Can you work these out from the drawing? Everything is in mm from the part's minimum corner. A direction names the side the tool comes from. Round coordinates to 2 decimals unless told otherwise and drop trailing zeros. Order: outer loops, then holes, each group sorted by start corner. A loop starts at its lowest first (then second) coordinate and runs counter-clockwise, first axis right, second up. Notation, with made-up numbers: (42.5, 17) -> (96.5, 17) arc R17 ccw to (96.5, 32) -> close; hole circle Ø7 at (15.25, 86.5). An arc over 180 degrees is marked (long way). One line per item, written item: value.
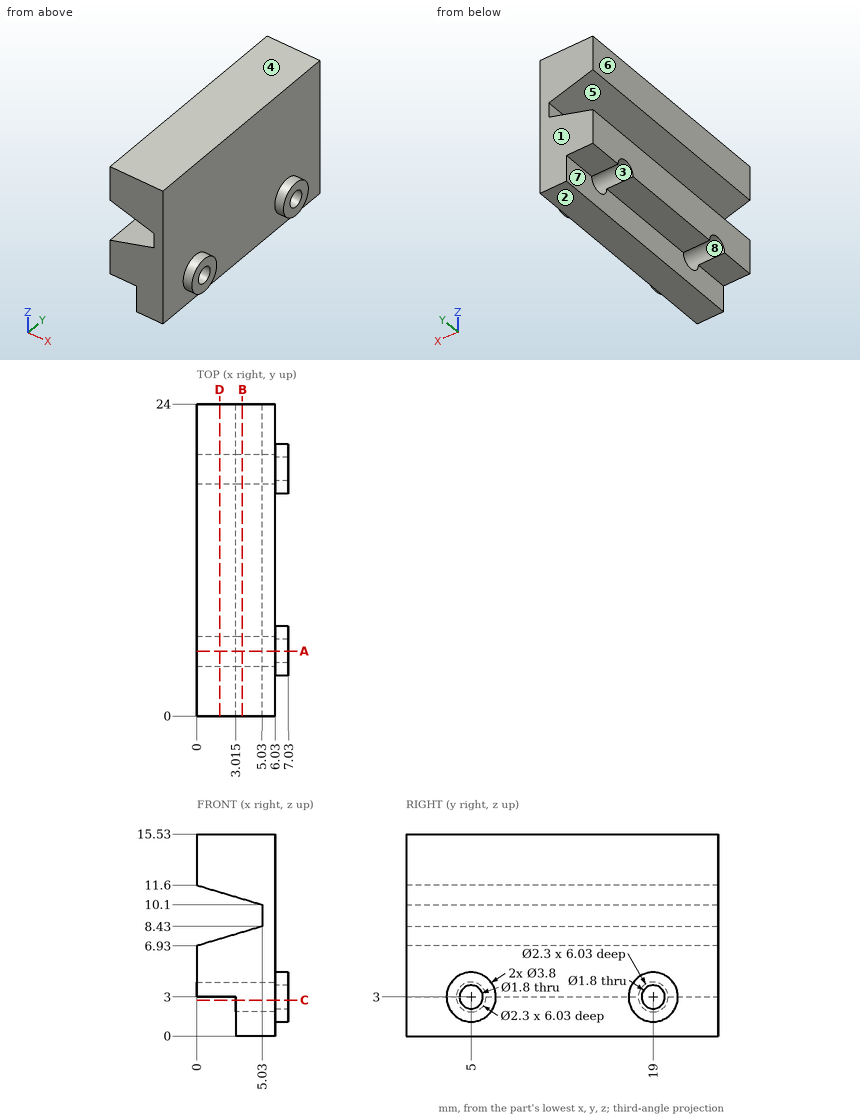
Q1. On a 3-axis mill with a long thin cutter (end or side, diameter ignored), from which of +Z, -Z, +X, -X, +Y, -Y can I reach the whole of each face in a straight line? I mean the marked faces 5, 6, 7 and 8. Say none if no direction works.
Answers below:
face 5: -X, +Y, -Y
face 6: +Z, -Z, -X, +Y, -Y
face 7: -Z, -X, +Y, -Y
face 8: -X
Q2. Will these pins go through, and if not, where does the flat tip stop? pin 1 Ø2 at (y, z) = (19, 3) entering from -X; pin 2 Ø1.4 at (y, z) = (5, 3) entering from -X; pin 3 Ø2.5 at (x, y) = (1, 1) entering from -Z; pin 4 Ø2.5 at (y, z) = (8, 1) entering from -X (3 decimals).
Answers below:
pin 1: x = 6.03
pin 2: through
pin 3: z = 3
pin 4: x = 3.015
Q3. I want a section at C-C on z = 2.75. Give the number of separate pieces and of enclosed holes in the cut face, plus the area to 3 significant figures.
Answers below:
separate pieces: 3
enclosed holes: 0
area: 62.9 mm^2
Q4. I want a section at B-B on x = 3.5. List the corners of the cut face in (y, z) for me.
Answers below:
outline: (0, 0) -> (24, 0) -> (24, 7.97) -> (0, 7.97) -> close; (0, 10.56) -> (24, 10.56) -> (24, 15.53) -> (0, 15.53) -> close; hole circle Ø2.3 at (5, 3); hole circle Ø2.3 at (19, 3)
Q5. I want a section at D-D on x = 1.75. List the corners of the cut face in (y, z) for me.
Answers below:
outline: (0, 3) -> (3.85, 3) arc R1.15 cw to (6.15, 3) -> (17.85, 3) arc R1.15 cw to (20.15, 3) -> (24, 3) -> (24, 7.45) -> (0, 7.45) -> close; (0, 11.08) -> (24, 11.08) -> (24, 15.53) -> (0, 15.53) -> close
Q6. Please list where these lines run through material, in increasing order: line 1 along Y through (x, z) = (6.7, 3); line 2 along Y through (x, z) = (4.5, 2); line 3 along X through (y, z) = (19.5, 12.75).
Answers below:
line 1: 3.1 to 4.1, 5.9 to 6.9, 17.1 to 18.1, 19.9 to 20.9
line 2: 0 to 4.43, 5.57 to 18.43, 19.57 to 24
line 3: 0 to 6.03
Q7. We'd pull the mould along Z, two halves only. Please class the marked faces 1, 2, 3 and 4: released by +Z, released by -Z, zero draft, split by the parting line, or undercut.
Answers below:
face 1: zero draft
face 2: released by -Z
face 3: undercut
face 4: released by +Z
Q8. I want a section at A-A on y = 5. List the corners of the cut face in (x, z) for me (3 decimals), plus the area to 3 significant figures.
Answers below:
outline: (0, 4.15) -> (6.03, 4.15) -> (6.03, 3.9) -> (7.03, 3.9) -> (7.03, 4.9) -> (6.03, 4.9) -> (6.03, 15.53) -> (0, 15.53) -> (0, 11.6) -> (5.03, 10.1) -> (5.03, 8.43) -> (0, 6.93) -> close; (3.015, 0) -> (6.03, 0) -> (6.03, 1.1) -> (7.03, 1.1) -> (7.03, 2.1) -> (6.03, 2.1) -> (6.03, 1.85) -> (3.015, 1.85) -> close
area: 60.3 mm^2
